from build123d import *

# Parameters (mm, degrees)
SKETCH_1_W          = 20
SKETCH_1_H          = 45
EXTRUDE_1_DEPTH     = 15
SKETCH_4_W          = 11
SKETCH_4_H          = 20
EXTRUDE_2_DEPTH     = 16
CUT_EXTRUDE_1_DEPTH = 11.4


with BuildPart() as part:
    # 草图1 → 凸台-拉伸1 (new body)
    with BuildSketch(Plane(origin=(0, 0, 0), x_dir=(0, 0, -1), z_dir=(1, 0, 0))):
        with Locations((-10, 0)):
            Rectangle(SKETCH_1_W, SKETCH_1_H)
    extrude(amount=EXTRUDE_1_DEPTH)

    # 草图4 → 凸台-拉伸2 (add)
    with BuildSketch(Plane(origin=(0, 0, 0), x_dir=(0, 0, -1), z_dir=(1, 0, 0))):
        with Locations((-25.5, 0)):
            Rectangle(SKETCH_4_W, SKETCH_4_H)
    extrude(amount=EXTRUDE_2_DEPTH)

    # 草图2 → 切除-拉伸1 (cut)
    with BuildSketch(Plane(origin=(0, 0, 0), x_dir=(0, 0, -1), z_dir=(1, 0, 0))):
        with BuildLine():
            Line((-17.9, 13.1), (-17.9, -13.1))
            ThreePointArc((-17.9, -13.1), (-10, -21), (-2.1, -13.1))
            Line((-2.1, -13.1), (-2.1, 13.1))
            ThreePointArc((-2.1, 13.1), (-10, 21), (-17.9, 13.1))
        make_face()
    extrude(amount=CUT_EXTRUDE_1_DEPTH, mode=Mode.SUBTRACT)


solid = part.part
Input: part model. Units: mm. Frame: model coordinates. A direction names the side the tool comes from. Give positions to 0.01 mm unless a question says otherwise; leave off trailing zeros. Write each loop counter-clockwise with the first axis right and the second up, starting at its lowest first coordinate (ties: lowest second). Pieces come first, ordered by that corner, then holes.
Q1. Section C-C, the plane z = 10. Output: boundary loops of the cut face in (x, y).
Q2. First-contact query: P1, Ø0.8, axis at x = 15.5, y = 4, coming from the -Z side; P2, Ø4, axis at x = 6, y = -19, coming from the +Z side; P3, Ø8, axis at y = -4, z = 11, coming from the -X side. Flat tips, straight axial feed; report the tip coordinate or a pass-through.
Q3. Material intervals for probe 1 along Z at (x, y) = (1.5, 7); probe 2 along Z at (x, y) = (1.25, -11.5); probe 3 along Z at (x, y) = (14.25, -17.5), sorted ascending.
Q4. Set-up query: faces 4 (the face through (6, 21, 10)), 5 (the face through (8, 10, 26)), 6 (the face through (15.5, -0.1, 20)). Return all of +Z, -Z, +X, -X, +Y, -Y with unobstructed straight access to the full face (end or side cutting, diameter ignored); none if empty.
Q5. Section B-B, the plane y = 12. Output: boundary loops of the cut face in (x, z), plus the area to 3 significant figures.
Q6. Section A-A, the plane x = 9.75. Output: boundary loops of the cut face in (y, z).
Q7. Pull-direction query (Y, two-part tool) for faces 1 (the face through (6, -21, 10)), 2 (the face through (7, 16, 20)), 3 (the face through (8, -10, 26)); classes: pulls with the +Y half, pulls with the -Y half, needs draft (parallel to the pull), parting line crosses it, or undercut.
Q8. Section D-D, the plane z = 27.5. Output: boundary loops of the cut face in (x, y), plus the area to 3 significant figures.
Filled in:
1. outline: (0, -22.5) - (15, -22.5) - (15, 22.5) - (0, 22.5) - (0, 21) - (11.4, 21) - (11.4, -21) - (0, -21) - close
2. P1: stops at z = 20
2. P2: stops at z = 20
2. P3: stops at x = 11.4
3. probe 1: z = 0 to 2.1, 17.9 to 31
3. probe 2: z = 0 to 2.1, 17.9 to 20
3. probe 3: z = 0 to 20
4. face 4: -X
4. face 5: +Z, +X, -X, +Y
4. face 6: -Z, +X, +Y, -Y
5. outline: (0, 0) - (15, 0) - (15, 20) - (0, 20) - (0, 17.9) - (11.4, 17.9) - (11.4, 2.1) - (0, 2.1) - close
5. area: 120 mm2
6. outline: (-22.5, 0) - (22.5, 0) - (22.5, 20) - (10, 20) - (10, 31) - (-10, 31) - (-10, 20) - (-22.5, 20) - close; hole (-13.1, 2.1) - (13.1, 2.1) arc R7.9 ccw to (13.1, 17.9) - (-13.1, 17.9) arc R7.9 ccw to start
7. face 1: undercut
7. face 2: needs draft
7. face 3: pulls with the -Y half
8. outline: (0, -10) - (16, -10) - (16, 10) - (0, 10) - close
8. area: 320 mm2
